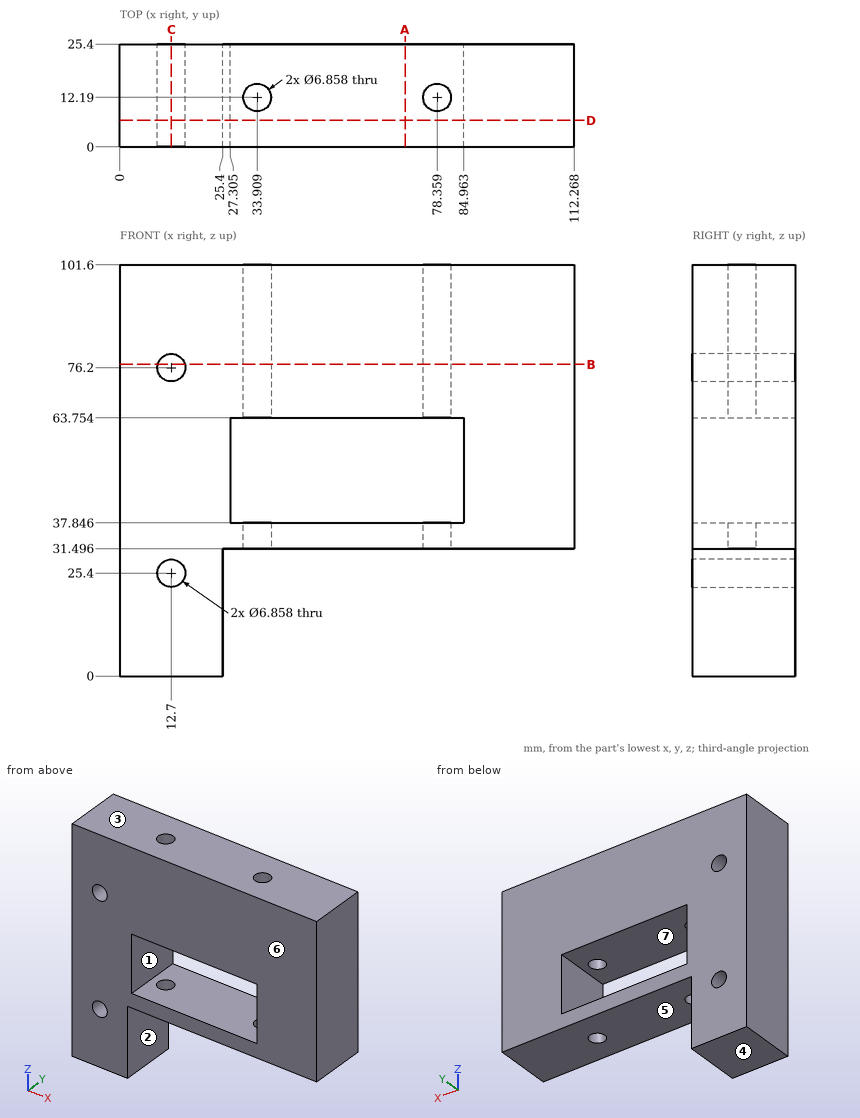
Drawing for the job (mm, zero at the part's lowest x, y, z). A direction names the side the tool comes from. Give positions to 0.01 mm unless a question says otherwise; leave off trailing zeros. Order: outer loops, then holes, each group sorted by start corner. A loop starts at its lowest first (then second) coordinate and runs counter-clockwise, first axis right, second up. Notation, with made-up numbers: (83, 8) - (92, 8) arc R30 cw to (92, 34) - close; hole circle Ø10 at (26.5, 38). An arc over 180 degrees is marked (long way). Use one line per item in the form item = value.
Item 1: Slice it at B-B on z = 77. Give the cut face in (x, y), and give its area (3 significant figures).
Solution:
outline = (0, 0) - (9.37, 0) - (9.37, 25.4) - (0, 25.4) - close; (16.03, 0) - (112.27, 0) - (112.27, 25.4) - (16.03, 25.4) - close; hole circle Ø6.86 at (33.91, 12.19); hole circle Ø6.86 at (78.36, 12.19)
area = 2,610 mm2
Item 2: Which spindle directions (+Z, -Z, +X, -X, +Y, -Y) get a long thin tool onto all of the face, cutting with end or side? Do the marked faces 5, 6 and 7. Say none if no direction does.
Solution:
face_5 = -Z, +X, +Y, -Y
face_6 = +Z, -Z, +X, -X, -Y
face_7 = +Y, -Y
Item 3: Two-plate mould, pull along Z, no slides. Class the marked faces 1, 2, 3 and 4: released by +Z, released by -Z, zero draft, split by the parting line, or undercut.
Solution:
face_1 = undercut
face_2 = zero draft
face_3 = released by +Z
face_4 = released by -Z
Item 4: Slice it at D-D on y = 6.5. Give the cut face in (x, z) (3 decimals).
Solution:
outline = (0, 0) - (25.4, 0) - (25.4, 31.496) - (112.268, 31.496) - (112.268, 101.6) - (0, 101.6) - close; hole circle Ø6.858 at (12.7, 25.4); hole circle Ø6.858 at (12.7, 76.2); hole (27.305, 37.846) - (84.963, 37.846) - (84.963, 63.754) - (27.305, 63.754) - close
Item 5: Probe probe 1 along X at (y, z) = (17.5, 52.5) (3 decimals); probe 2 along X at (y, z) = (6.75, 76.2); probe 3 along Z at (x, y) = (84, 15.25). List the from-to ranges inside material, lowest first. Write a range as from..to.
Solution:
probe_1 = 0..27.305, 84.963..112.268
probe_2 = 0..9.27, 16.13..112.27
probe_3 = 31.5..37.85, 63.75..101.6
Item 6: Slice it at A-A on x = 70.5. Give the cut face in (y, z).
Solution:
outline = (0, 31.5) - (25.4, 31.5) - (25.4, 37.85) - (0, 37.85) - close; (0, 63.75) - (25.4, 63.75) - (25.4, 101.6) - (0, 101.6) - close
Item 7: Slice it at C-C on x = 12.7. Give the cut face in (y, z), and give its area (3 significant figures).
Solution:
outline = (0, 0) - (25.4, 0) - (25.4, 21.97) - (0, 21.97) - close; (0, 28.83) - (25.4, 28.83) - (25.4, 72.77) - (0, 72.77) - close; (0, 79.63) - (25.4, 79.63) - (25.4, 101.6) - (0, 101.6) - close
area = 2,230 mm2
Item 8: Pin check, flat tip, straight feed: pin 1 Ø12.5 at (y, z) = (9, 14.5) entering from +X. Stop position of the tip, or through.
Solution:
pin_1 = 25.4
